Input: part model. Units: mm. Frame: model coordinates. A direction names the side the tool comes from. Give positions to 0.01 mm unless a question says otherwise; leave off trailing zeros. Loops run counter-clockwise (first coordinate to the right, second up) from the corner with the lowest first, then second, coordinate; pieces in that order, holes last. Notation, with made-up numbers: M -39,26.25 L -4,26.25 A10 ccw -4,39.25 Z; hole C 86,-36.5 d4. An arc over 180 degrees is marked long. Answer as a JSON object with one key per item and string values. Group by question number.
Autodesk Fusion 360 part; units mm, degrees
sketch "Sketch1" plane through (0, 0, 0) normal (0, 0, 1) x (1, 0, 0)
  line L0 (24, 9.5) -> (24, -22)
  line L1 (23, -23) -> (-9, -23)
  line L2 (-10.5, -22) -> (-10.5, 9.5)
  line L3 (-11.5, 10.5) -> (25, 10.5)
  line L4 (25, 10.5) -> (25, 9.5)
  line L5 (-11.5, 9.5) -> (-11.5, 10.5)
  line L6 (-11.5, 9.5) -> (-10.5, 9.5)
  line L7 (24, 9.5) -> (25, 9.5)
  line L8 (-10.5, -22) -> (-10.5, -23)
  line L9 (-10.5, -23) -> (-9, -23)
  line L10 (23, -23) -> (24, -23)
  line L11 (24, -23) -> (24, -22)
  point P0 (24, -23)
  point P1 (-10.5, -23)
  dimension "d3" = 1
  dimension "d4" = 33.5
  dimension "d5" = 1
  dimension "d6" = 34.5
  dimension "d32" = 1
extrude "Extrude3" add sketch "Sketch1" along normal blind 2
sketch "Sketch7" plane through (0, 0, 2) normal (0, 0, 1) x (-1, 0, 0)
  line L0 (10.5, 23) -> (-24, 23)
  line L1 (-24, 23) -> (-24, -9.5)
  line L2 (-24, -9.5) -> (-25, -9.5)
  line L3 (-25, -9.5) -> (-25, -10.5)
  line L4 (-25, -10.5) -> (11.5, -10.5)
  line L5 (11.5, -10.5) -> (11.5, -9.5)
  line L6 (11.5, -9.5) -> (10.5, -9.5)
  line L7 (10.5, -9.5) -> (10.5, 23)
  line L8 (10.5, -9.5) -> (8.5, -9.5)
  line L9 (8.5, -9.5) -> (8.5, 8.0024)
  line L10 (8.5, 8.0024) -> (10.5, 8.0024)
  line L11 (10.5, 8.0024) -> (10.5, -9.5)
  line L12 (-24, -9.5) -> (-22, -9.5)
  line L13 (-22, -9.5) -> (-22, 8)
  line L14 (-22, 8) -> (-24, 8)
  line L15 (-24, 8) -> (-24, -9.5)
  dimension "d26" = 2
  dimension "d27" = 2
extrude "Extrude4" cut sketch "Sketch7" against normal blind 2 contours L7 L8 L9 L10 L11 | L1 L12 L13 L14 L15
extrude "Extrude5" cut 1 faces at (1.6667, -2.1675, 2) along direction (0, 0, -1) blind 1
1. Reachability of faces 1 (the flat face through (-10, 9.5, 0.5)), 2 (the flat face through (24, -15.4, 0.5)), 3 (the flat face through (22, 0.9, 0.5)) from +Z, -Z, +X, -X, +Y, -Y: full face, straight path, thin tool, end or side. Return the list, or none.
2. Section C-C (y = -13). Output: boundary loops of the cut face in (x, z).
3. Section A-A (z = 0.85). Output: boundary loops of the cut face in (x, y).
4. Material intervals for L1, parallel to X at y = 8, z = 0.3; L2, parallel to Y at x = 23.5, z = 0.45; L3, parallel to X at y = -10, z = 0.25, sorted ascending.
5. Section B-B (y = -4.5). Output: boundary loops of the cut face in (x, z).
6. Mould query, pull axis Y, two halves, no side actions, for faces 4 (the flat face through (23, -8, 0.5)), 5 (the flat face through (6.5, -23, 0.5)), 6 (the flat face through (6.5, 10.5, 0.5)), 7 (the flat face through (6, -6, 1)). Classes: pulls with the +Y half, pulls with the -Y half, needs draft (parallel to the pull), parting line crosses it, or undercut.
7. First-contact query: P1, Ø2, axis at x = 3, y = -2, coming from the -Z side. Flat tip, straight axial feed; report the tip coordinate or a pass-through.
Geometry results:
{
 "1": {"face 1": "+Z, -Z, -X", "face 2": "+Z, -Z, +X, -Y", "face 3": "+Z, -Z, +X"},
 "2": {"outline": "M -10.5,0 L 24,0 L 24,1 L -10.5,1 Z"},
 "3": {"outline": "M -11.5,9.5 L -8.5,9.5 L -8.5,-8 L -10.5,-8 L -10.5,-23 L 24,-23 L 24,-8 L 22,-8 L 22,9.5 L 25,9.5 L 25,10.5 L -11.5,10.5 Z"},
 "4": {"L1": "-8.5 to 22", "L2": "-23 to -8, 9.5 to 10.5", "L3": "-10.5 to 24"},
 "5": {"outline": "M -8.5,0 L 22,0 L 22,1 L -8.5,1 Z"},
 "6": {"face 4": "undercut", "face 5": "pulls with the -Y half", "face 6": "pulls with the +Y half", "face 7": "needs draft"},
 "7": {"P1": "z = 0"}
}
